Part print with two shaded views. Sizes in mm from the minimum x, y, z corner. A direction names the side the tool comes from. Give positions to 0.01 mm unless a question says otherwise; leave off trailing zeros. Write each loop counter-clockwise with the first axis right and the second up, starting at its lowest first coordinate (ties: lowest second). Pieces come first, ordered by that corner, then holes.
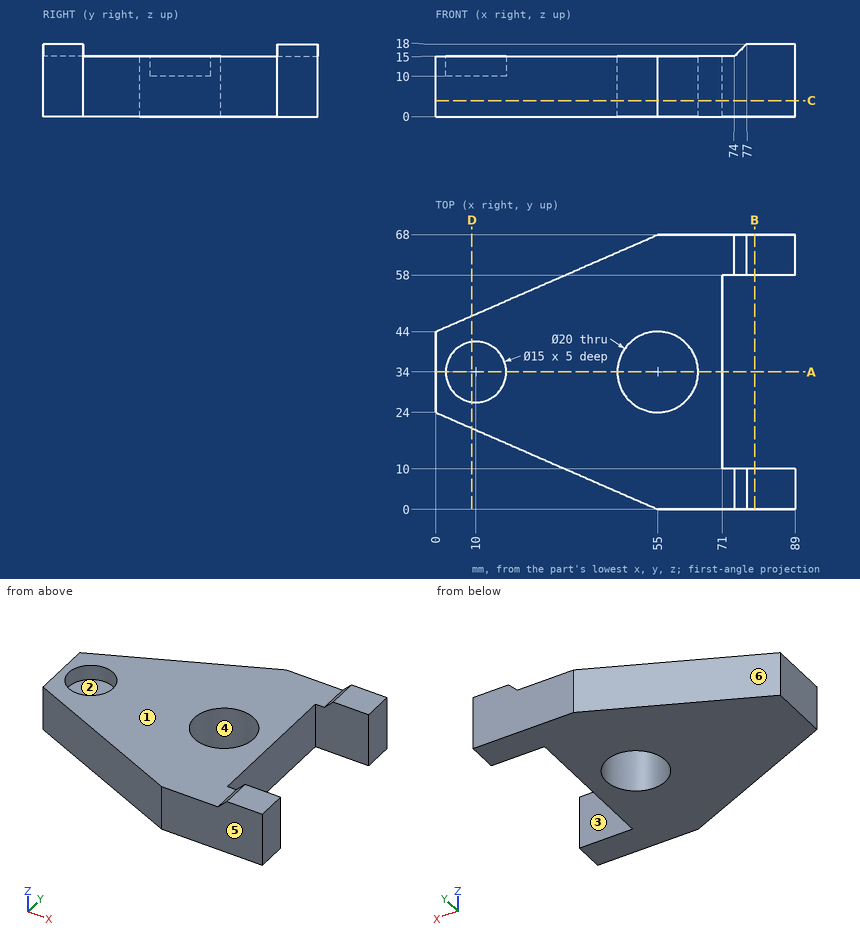
1) Wall check: L1, parallel to Y at x = 84.5, z = 7.5; L2, parallel to Y at x = 55, z = 5; L3, parallel to X at y = 34, z = 9.5. Give the ranges that are in metal, low to high.
Answers follow:
L1: y = 0 to 10, 58 to 68
L2: y = 0 to 24, 44 to 68
L3: x = 0 to 45, 65 to 71
2) 3-axis set-ups, long thin cutter, end or side, ignore diameter. For the marked faces 1, 2 and 3: which of +Z, -Z, +X, -X, +Y, -Y reach the whole face in a straight line?
Answers follow:
face 1: +Z, -X, +Y, -Y
face 2: +Z
face 3: +Z, -Z, +X
3) Saw through at D-D, the plane x = 9. Write the cut outline in (y, z).
Answers follow:
outline: (20.07, 0) - (47.93, 0) - (47.93, 15) - (41.43, 15) - (41.43, 10) - (26.57, 10) - (26.57, 15) - (20.07, 15) - close
4) Two-plate mould, pull along X, no slides. Class the marked faces 4, 5 and 6: +X half, -X half, draft (parallel to the pull), parting line (faces both ways), or undercut.
Answers follow:
face 4: undercut
face 5: draft
face 6: -X half
5) Saw through at B-B, the plane x = 79. Write the cut outline in (y, z), then the cut area to 3 significant figures.
Answers follow:
outline: (0, 0) - (10, 0) - (10, 18) - (0, 18) - close; (58, 0) - (68, 0) - (68, 18) - (58, 18) - close
area: 360 mm2
6) Saw through at C-C, the plane z = 4. Write the cut outline in (x, y), then the cut area to 3 significant figures.
Answers follow:
outline: (0, 24) - (55, 0) - (89, 0) - (89, 10) - (71, 10) - (71, 58) - (89, 58) - (89, 68) - (55, 68) - (0, 44) - close; hole circle Ø20 at (55, 34)
area: 3,550 mm2
7) Saw through at A-A, the plane y = 34. Write the cut outline in (x, z), then the cut area to 3 significant figures.
Answers follow:
outline: (0, 0) - (45, 0) - (45, 15) - (17.5, 15) - (17.5, 10) - (2.5, 10) - (2.5, 15) - (0, 15) - close; (65, 0) - (71, 0) - (71, 15) - (65, 15) - close
area: 690 mm2
8) Pin check, flat tips, straight feed: pin 1 Ø4 at (x, z) = (9.5, 13) entering from +Y; pin 2 Ø8 at (x, z) = (33.5, 2.5) entering from +Y; pin 3 Ø16.5 at (x, y) = (8, 34.5) entering from +Z. Stop position of each tip, or through.
Answers follow:
pin 1: stops at y = 49.02
pin 2: stops at y = 60.36
pin 3: stops at z = 15
